```python
from build123d import *
from build123d.topology import SkipClean

# Parameters (mm, degrees)
SKETCH1_R           = 0.5
SKETCH1_R_2         = 1.5
BOSS_EXTRUDE3_DEPTH = 1.5
SKETCH2_R           = 3.5
BOSS_EXTRUDE4_DEPTH = 3
BOSS_EXTRUDE5_START = 0.5
SKETCH3_R           = 3.5
SKETCH3_R_2         = 3.25
BOSS_EXTRUDE5_DEPTH = 0.5
SKETCH4_R           = 2.75
CUT_EXTRUDE1_DEPTH  = 4


with BuildPart() as part:
    # Sketch1 → Boss-Extrude3 (new body)
    with BuildSketch(Plane.XY):
        with BuildLine():
            Line((-3.4, 0.830662386), (-1.681759988, 13.206282347))
            ThreePointArc((-1.681759988, 13.206282347), (-1.181043929, 14.131243458), (-0.196011829, 14.5))
            Line((-0.196011829, 14.5), (0.196011829, 14.5))
            ThreePointArc((0.196011829, 14.5), (1.181043929, 14.131243458), (1.681759988, 13.206282347))
            Line((1.681759988, 13.206282347), (3.4, 0.830662386))
            ThreePointArc((3.4, 0.830662386), (3.5, 0), (3.4, -0.830662386))
            Line((3.4, -0.830662386), (1.681759988, -13.206282347))
            ThreePointArc((1.681759988, -13.206282347), (1.181043929, -14.131243458), (0.196011829, -14.5))
            Line((0.196011829, -14.5), (-0.196011829, -14.5))
            ThreePointArc((-0.196011829, -14.5), (-1.181043929, -14.131243458), (-1.681759988, -13.206282347))
            Line((-1.681759988, -13.206282347), (-3.4, -0.830662386))
            ThreePointArc((-3.4, -0.830662386), (-3.5, 0), (-3.4, 0.830662386))
        make_face()
        with Locations((0, 10)):
            Circle(SKETCH1_R, mode=Mode.SUBTRACT)
        with Locations((0, 12.5)):
            Circle(SKETCH1_R, mode=Mode.SUBTRACT)
        with Locations((0, 7.5)):
            Circle(SKETCH1_R, mode=Mode.SUBTRACT)
        Circle(SKETCH1_R_2, mode=Mode.SUBTRACT)
        with Locations(Location((0, -7.5, 0), (0, 0, 180))):
            Circle(SKETCH1_R, mode=Mode.SUBTRACT)
        with Locations(Location((0, -12.5, 0), (0, 0, 180))):
            Circle(SKETCH1_R, mode=Mode.SUBTRACT)
        with Locations(Location((0, -10, 0), (0, 0, 180))):
            Circle(SKETCH1_R, mode=Mode.SUBTRACT)
    extrude(amount=BOSS_EXTRUDE3_DEPTH)

    # Sketch2 → Boss-Extrude4 (add)
    with SkipClean():  # the faces are left unmerged after this step: merging them gives an invalid solid
        with BuildSketch(Plane.XY.offset(1.5)):
            with Locations(Location((0, 0, 0), (0, 0, 166.270867325))):
                Circle(SKETCH2_R)
        extrude(amount=BOSS_EXTRUDE4_DEPTH)

    # Sketch3 → Boss-Extrude5 (add)
    with SkipClean():  # the faces are left unmerged after this step: merging them gives an invalid solid
        with BuildSketch(Plane(origin=(0, 0, 0), x_dir=(-1, 0, 0), z_dir=(0, 0, -1)).offset(BOSS_EXTRUDE5_START)):
            Circle(SKETCH3_R)
            Circle(SKETCH3_R_2, mode=Mode.SUBTRACT)
        extrude(amount=-BOSS_EXTRUDE5_DEPTH)

    # Sketch4 → Cut-Extrude1 (cut)
    with SkipClean():  # the faces are left unmerged after this step: merging them gives an invalid solid
        with BuildSketch(Plane.XY.offset(4.5)):
            Circle(SKETCH4_R)
        extrude(amount=-CUT_EXTRUDE1_DEPTH, mode=Mode.SUBTRACT)


solid = part.part
```
Geometry check sheet. Reference: the model listing, model coordinates, mm. A direction names the side the tool comes from. Round coordinates to 2 decimals unless told otherwise and drop trailing zeros. Loops run counter-clockwise (first coordinate to the right, second up) from the corner with the lowest first, then second, coordinate; pieces in that order, holes last. Notation, with made-up numbers: (-6.5, -11) - (14.5, -11) arc R10 cw to (14.5, -1) - close; hole circle Ø9 at (58.5, 46.25). An arc over 180 degrees is marked (long way). Write item = value, one per line. Start each with the question number.
1. Section check B-B on x = 3. Enter the section's corners in (y, z).
2. Section check A-A on y = 0. Enter the section's corners in (x, z).
3. Section check C-C on z = 3.65. Enter the section's corners in (x, y).
4. Depth check by flat-ended pin: pin 1 (1 mm diameter, centred on x = -0.5, z = 1.5, fed in from -Y); pin 2 (3.5 mm diameter, centred on x = 0.5, y = -7.5, fed in from -Z); pin 3 (2 mm diameter, centred on x = -1, y = 4.5, fed in from +Z); pin 4 (3 mm diameter, centred on x = -1, y = -0.5, fed in from +Z). Enter the tip coordinate at first touch or a pass-through.
5. Mould release check, pull along X, two halves, no side actions. Record for faces 1 (the face through (-2.53, -7.11, 0.74)), 2 (the face through (-0.596, -2.685, 2.528)), 3 (the face through (1, 8, 1.5)): released by +X, released by -X, zero draft, split by the parting line, or undercut.
6. Set-up check for faces 4 (the face through (2.553, -6.932, 0.74)), 5 (the face through (1.2, -1.2, 0.5)), 6 (the face through (-0.7, 1.5, 0)): record each of +Z, -Z, +X, -X, +Y, -Y from which the full face is reachable in a straight line by a thin tool's end or side.
7. Thickness scan on line 1 (Y direction, x = 0, z = 1.75); line 2 (Z direction, x = 0, y = 6.75); line 3 (Z direction, x = 1, y = 2.25). Record the ranges inside material, lowest first.
8. Section check D-D on y = 10. Enter the section's corners in (x, z).
Working result:
q1.outline = (-3.71, 0) - (-1.8, 0) - (-1.8, -0.5) - (-1.25, -0.5) - (-1.25, 0) - (1.25, 0) - (1.25, -0.5) - (1.8, -0.5) - (1.8, 0) - (3.71, 0) - (3.71, 1.5) - (1.8, 1.5) - (1.8, 4.5) - (-1.8, 4.5) - (-1.8, 1.5) - (-3.71, 1.5) - close
q2.outline = (-3.5, -0.5) - (-3.25, -0.5) - (-3.25, 0) - (-1.5, 0) - (-1.5, 0.5) - (-2.75, 0.5) - (-2.75, 4.5) - (-3.5, 4.5) - close; (1.5, 0) - (3.25, 0) - (3.25, -0.5) - (3.5, -0.5) - (3.5, 4.5) - (2.75, 4.5) - (2.75, 0.5) - (1.5, 0.5) - close
q3.outline = circle Ø7 at (0, 0); hole circle Ø5.5 at (0, 0)
q4.pin_1 = -14.5
q4.pin_2 = 0
q4.pin_3 = 1.5
q4.pin_4 = 0.5
q5.face_1 = released by -X
q5.face_2 = undercut
q5.face_3 = zero draft
q6.face_4 = +Z, -Z, +X, -Y
q6.face_5 = +Z
q6.face_6 = -Z
q7.line_1 = -3.5 to -2.75, 2.75 to 3.5
q7.line_2 = 0 to 1.5
q7.line_3 = 0 to 0.5
q8.outline = (-2.13, 0) - (-0.5, 0) - (-0.5, 1.5) - (-2.13, 1.5) - close; (0.5, 0) - (2.13, 0) - (2.13, 1.5) - (0.5, 1.5) - close
